Can you work these out from the model? Positions are in its coordinate system, mm. A direction names the side the tool comes from. Give positions to 0.01 mm unless a question says otherwise; leave off trailing zeros. Loops run counter-clockwise (first coordinate to the right, second up) from the corner with the lowest first, then second, coordinate; pieces in that order, holes last. Notation, with made-up numbers: M -11,-9 L 43,-9 A23 cw 43,22 Z; hole C -35.5,-7 d11. An arc over 180 degrees is marked long. Answer as a JSON object with one key per item and string values.
```python
from build123d import *

# Parameters (mm, degrees)
F1_DEPTH = 150
F3_D     = 8
F3_DEPTH = 7
F3_TIP   = 2.4034424761
F5_DEPTH = 6.1


with BuildPart() as f1:
    # F0 (on Top) → F1 (new body)
    with BuildSketch(Plane.XY):
        with BuildLine():
            Line((37.5, 0), (-37.5, 0))
            Line((-37.5, 0), (-37.5, -40))
            Line((-37.5, -40), (-31.4, -40))
            Line((-31.4, -40), (-31.4, -11.8))
            ThreePointArc((-31.4, -11.8), (-29.0568542495, -6.1431457505), (-23.4, -3.8))
            Line((-23.4, -3.8), (23.4, -3.8))
            ThreePointArc((23.4, -3.8), (29.0568542495, -6.1431457505), (31.4, -11.8))
            Line((31.4, -11.8), (31.4, -40))
            Line((31.4, -40), (37.5, -40))
            Line((37.5, -40), (37.5, 0))
        make_face()
    extrude(amount=F1_DEPTH)

    # F3
    with Locations(Plane.YZ.offset(37.5)):
        with Locations((-20, 114), (-20, 36)):
            Hole(F3_D / 2, depth=F3_DEPTH)
            with Locations((0, 0, -(F3_DEPTH + F3_TIP / 2))):  # 118° drill point
                Cone(0, F3_D / 2, F3_TIP, mode=Mode.SUBTRACT)

    # F4 (on face) → F5 (cut, through all)
    with BuildSketch(Plane(origin=(-37.5, 0, 0), x_dir=(0, -1, 0), z_dir=(-1, 0, 0))):
        with BuildLine():
            Line((24, 106), (24, 138))
            ThreePointArc((24, 138), (20, 142), (16, 138))
            Line((16, 138), (16, 106))
            ThreePointArc((16, 106), (20, 110), (24, 106))
        make_face()
        with BuildLine():
            ThreePointArc((16, 106), (20, 102), (24, 106))
            ThreePointArc((24, 106), (20, 110), (16, 106))
        make_face()
        with BuildLine():
            ThreePointArc((16.0041883178, 43.817), (20.0915239614, 40.0010472165), (24, 44))
            ThreePointArc((24, 44), (20.0915239614, 47.9989527835), (16.0041883178, 44.183))
            Line((16.0041883178, 44.183), (16.0041883178, 43.817))
        make_face()
        with BuildLine():
            Line((16.0041883178, 12.183), (16.0041883178, 11.817))
            ThreePointArc((16.0041883178, 11.817), (20.0915239614, 8.0010472165), (24, 12))
            ThreePointArc((24, 12), (20.0915239614, 15.9989527835), (16.0041883178, 12.183))
        make_face()
        with BuildLine():
            ThreePointArc((16.0041883178, 12.183), (20.0915239614, 15.9989527835), (24, 12))
            Line((24, 12), (24, 44))
            ThreePointArc((24, 44), (20.0915239614, 40.0010472165), (16.0041883178, 43.817))
            Line((16.0041883178, 43.817), (16.0041883178, 12.183))
        make_face()
    extrude(amount=-F5_DEPTH, mode=Mode.SUBTRACT)


solid = f1.part
```
1) Suppose I cut it at D-D, the plane z = 72.5. Write out the boundary of the cut face in (x, y).
Answer list:
{"outline": "M -37.5,-40 L -31.4,-40 L -31.4,-11.8 A8 cw -23.4,-3.8 L 23.4,-3.8 A8 cw 31.4,-11.8 L 31.4,-40 L 37.5,-40 L 37.5,0 L -37.5,0 Z"}
2) If we mould it in two halves opening along Z, with no side actions, what happens to faces 4 (the cylindrical face through (-34, -20, 102)), 5 (the flat face through (2.6, -3.6, 0)), 6 (the flat face through (2.6, -3.6, 150)), 7 (the cylindrical face through (-29.119, -6.206, 73.95))? For each: +Z half, -Z half, draft (parallel to the pull), parting line (faces both ways), or undercut.
Answer list:
{"face 4": "undercut", "face 5": "-Z half", "face 6": "+Z half", "face 7": "draft"}
3) Please list where these lines run through material, in increasing order: line 1 along Z through (x, y) = (34, -20); line 2 along X through (y, z) = (-28, 62); line 3 along Y through (x, z) = (-32, 127.5). Write a range as from..to.
Answer list:
{"line 1": "0..32, 40..110, 118..150", "line 2": "-37.5..-31.4, 31.4..37.5", "line 3": "-40..-24, -16..0"}
4) For faces 1 (the cylindrical face through (-34, -20, 142)), 2 (the flat face through (-31.4, -26, 74)), 3 (the cylindrical face through (34.407, -19.479, 39.966)), which set-ups out of +Z, -Z, +X, -X, +Y, -Y let a thin tool reach every point of the face, with its end or its side?
Answer list:
{"face 1": "-X", "face 2": "+Z, -Z, -Y", "face 3": "+X, -X"}
5) Suppose I cut it at C-C, the plane z = 114. Write out the boundary of the cut face in (x, y), and give its area (3 significant figures).
Answer list:
{"outline": "M -37.5,-40 L -31.4,-40 L -31.4,-24 L -37.5,-24 Z; M -37.5,-16 L -31.4,-16 L -31.4,-11.8 A8 cw -23.4,-3.8 L 23.4,-3.8 A8 cw 31.4,-11.8 L 31.4,-16 L 37.5,-16 L 37.5,0 L -37.5,0 Z; M 31.4,-40 L 37.5,-40 L 37.5,-24 L 31.4,-24 Z", "area": "657 mm^2"}
6) Suppose I cut it at B-B, the plane y = -8. Write out the boundary of the cut face in (x, z).
Answer list:
{"outline": "M -37.5,0 L -30.44,0 L -30.44,150 L -37.5,150 Z; M 30.44,0 L 37.5,0 L 37.5,150 L 30.44,150 Z"}
7) Suppose I cut it at A-A, the plane z = 22. Write out the boundary of the cut face in (x, y).
Answer list:
{"outline": "M -37.5,-40 L -31.4,-40 L -31.4,-24 L -37.5,-24 Z; M -37.5,-16 L -31.4,-16 L -31.4,-11.8 A8 cw -23.4,-3.8 L 23.4,-3.8 A8 cw 31.4,-11.8 L 31.4,-40 L 37.5,-40 L 37.5,0 L -37.5,0 Z"}
8) Will this pin go through, and if not, where does the flat tip stop? pin 1 Ø8 at (x, z) = (-1.5, 132.5) entering from -Y.
Answer list:
{"pin 1": "y = -3.8"}
